Can you work these out from the model? Positions are in its coordinate system, mm. Give positions to 0.01 mm unless a question says otherwise; leave off trailing zeros. Loops run counter-clockwise (first coordinate to the right, second up) from the corner with the lowest first, then second, coordinate; pieces in that order, holes last. Notation, with made-up numbers: M 75.25,52 L 93.25,52 A19 cw 93.25,81 Z; hole C 16,-15.5 d11. An arc over 180 degrees is marked long. Use CSV: the item, a comma, the result in double quotes.
from build123d import *

# Parameters (mm, degrees)
SKETCH_1_W      = 10
SKETCH_1_H      = 10
SKETCH_1_R      = 1.5
EXTRUDE_1_DEPTH = 44
FILLET_1_R      = 4


with BuildPart() as part:
    # 草图1 → 凸台-拉伸1 (new body)
    with BuildSketch(Plane.XY):
        with Locations((-1.28, 2.34)):
            Rectangle(SKETCH_1_W, SKETCH_1_H)
        with Locations((-1.28, 2.34)):
            Circle(SKETCH_1_R, mode=Mode.SUBTRACT)
    extrude(amount=EXTRUDE_1_DEPTH)

    # 圆角1
    fillet_1_edges = [part.edges().sort_by_distance(p)[0] for p in [
        (3.72, -2.66, 22),
        (-6.28, -2.66, 22),
        (-6.28, 7.34, 22),
        (3.72, 7.34, 22),
    ]]
    fillet(fillet_1_edges, radius=FILLET_1_R)


solid = part.part
Q1. If we mould it in two halves opening along X, with no side actions, what happens to faces 1 (the cylindrical face through (2.517, 6.199, 22.308)), 2 (the cylindrical face through (-5.139, -1.457, 22.308)), 3 (the flat face through (-1, 7.34, 22)), 4 (the cylindrical face through (-0.59, 1.01, 21.69))? For each: released by +X, released by -X, zero draft, split by the parting line, or undercut.
Model answer:
face 1,"released by +X"
face 2,"released by -X"
face 3,"zero draft"
face 4,"undercut"
Q2. I'm going to push flat-ended pins straight in: P1, Ø2.5, axis at x = -1.28, y = 2.34, coming from the -Z side; P2, Ø1, axis at x = 2.5, z = 35, coming from the +Y side. Where does each tip first touch, or does it pass through?
Model answer:
P1,"through"
P2,"y = 6.63"
Q3. I want a section at C-C, the plane x = -1.28. Please give me the cut outline in (y, z), then the cut area to 3 significant figures.
Model answer:
outline,"M -2.66,0 L 0.84,0 L 0.84,44 L -2.66,44 Z; M 3.84,0 L 7.34,0 L 7.34,44 L 3.84,44 Z"
area,"308 mm2"
Q4. I want a section at A-A, the plane y = 2.34. Please give me the cut outline in (x, z).
Model answer:
outline,"M -6.28,0 L -2.78,0 L -2.78,44 L -6.28,44 Z; M 0.22,0 L 3.72,0 L 3.72,44 L 0.22,44 Z"
Q5. I want a section at D-D, the plane y = 6.75. Please give me the cut outline in (x, z), then the cut area to 3 significant figures.
Model answer:
outline,"M -4.37,0 L 1.81,0 L 1.81,44 L -4.37,44 Z"
area,"272 mm2"
Q6. I want a section at B-B, the plane z = 8.5. Please give me the cut outline in (x, y), then the cut area to 3 significant figures.
Model answer:
outline,"M -6.28,1.34 A4 ccw -2.28,-2.66 L -0.28,-2.66 A4 ccw 3.72,1.34 L 3.72,3.34 A4 ccw -0.28,7.34 L -2.28,7.34 A4 ccw -6.28,3.34 Z; hole C -1.28,2.34 d3"
area,"79.2 mm2"
Q7. Please list where these lines run through material, in increasing order: L1, parallel to Y at x = -1.28, z = 19.5; L2, parallel to X at y = 1, z = 10; L3, parallel to Y at x = -1.75, z = 24.5. Write a range as from..to.
Model answer:
L1,"-2.66..0.84, 3.84..7.34"
L2,"-6.27..-1.95, -0.61..3.71"
L3,"-2.66..0.92, 3.76..7.34"
